Autodesk Fusion 360 part; units mm, degrees
sketch "Sketch1" plane through (0, 0, 0) normal (0, 1, 0) x (1, 0, 0)
  circle A0 centre (0, 0) radius 10.5
  dimension "d1" = 21
extrude "Extrude1" add sketch "Sketch1" along normal blind 4
sketch "Sketch2" plane through (0, 4, 0) normal (0, 1, 0) x (-1, 0, 0)
  circle A0 centre (0, 0) radius 10.5
  circle A1 centre (0, 0) radius 1.5
  dimension "d4" = 3
extrude "Extrude2" cut sketch "Sketch2" against normal blind 0.5 contours A1
sketch "Sketch3" plane through (0, 4, 0) normal (0, 1, 0) x (-1, 0, 0)
  circle A0 centre (0, 0) radius 1.5
  circle A1 centre (0, 0) radius 10.5
  circle A2 centre (0, 0) radius 9
  circle A3 centre (0, 0) radius 3.75
  dimension "d7" = 1.5
  dimension "d20" = 7.5
extrude "Extrude3" cut sketch "Sketch3" against normal blind 0.25
fillet "Fillet1" radius 0.1 1 edges at (-9.7894, 3.75, -3.797)
ref_plane "WorkPlane1" through (0, 0, 10.5) normal (0, 0, 1) x (1, 0, 0)
sketch "Sketch4" plane through (0, 0, 10.5) normal (0, 0, 1) x (1, 0, 0)
  line L0 (-1, 0) -> (1, 0)
  line L1 (1, 0) -> (1, 1.5)
  line L2 (1, 1.5) -> (-1, 1.5)
  line L3 (-1, 1.5) -> (-1, 0)
  line L4 (10.5, 0) -> (-10.5, 0)
  dimension "d12" = 1.5
  dimension "d13" = 2
extrude "Extrude4" cut sketch "Sketch4" against normal blind 0.5
sketch "Sketch5" plane through (0, 0, 10) normal (0, 0, 1) x (1, 0, 0)
  line L0 (1, 0) -> (1, 1.5)
  line L1 (1, 1.5) -> (-1, 1.5)
  line L2 (-1, 1.5) -> (-1, 0)
  line L3 (-1, 0) -> (1, 0)
  line L4 (9, 4) -> (-9, 4)
  line L5 (0, 1.5) -> (0, 0) construction
  line L6 (0, 0.75) -> (-1, 0.75) construction
  circle A0 centre (-0.5, 0.75) radius 0.25
  circle A1 centre (0.5, 0.75) radius 0.25
  dimension "d16" = 0.5
extrude "Extrude5" add sketch "Sketch5" along normal blind 2 contours A0 | A1
Part model, mm, in its own coordinate system. A direction names the side the tool comes from. Round coordinates to 2 decimals unless told otherwise and drop trailing zeros. Loops run counter-clockwise (first coordinate to the right, second up) from the corner with the lowest first, then second, coordinate; pieces in that order, holes last. Notation, with made-up numbers: (29, -27.75) - (40, -27.75) arc R13 ccw to (40, -14.75) - close; hole circle Ø5 at (21.25, 55.5). An arc over 180 degrees is marked (long way). Answer as a JSON object with one key per item and string values.
Item 1: Band-saw the part on B-B on x = 0. List the corners of the cut face in (y, z).
Output:
{"outline": "(0, -10.5) - (3.65, -10.5) arc R0.1 ccw to (3.75, -10.4) - (3.75, -9) - (4, -9) - (4, -3.75) - (3.75, -3.75) - (3.75, -1.5) - (3.5, -1.5) - (3.5, 1.5) - (3.75, 1.5) - (3.75, 3.75) - (4, 3.75) - (4, 9) - (3.75, 9) - (3.75, 10.4) arc R0.1 ccw to (3.65, 10.5) - (1.5, 10.5) - (1.5, 10) - (0, 10) - close"}
Item 2: Tool access for faces 1 (the face through (0, 3.5, 0)), 2 (the face through (0, 0, 0)), 3 (the face through (0, 1, 10)): list every direction of +Z, -Z, +X, -X, +Y, -Y with a clear straight run to the whole face (end or side of a thin tool).
Output:
{"face 1": "+Y", "face 2": "+Z, -Z, +X, -X, -Y", "face 3": "+Z"}
Item 3: Band-saw the part on A-A on y = 0.75. List the corners of the cut face in (x, z).
Output:
{"outline": "(-1, 10) - (-1, 10.45) arc R10.5 ccw (long way) to (1, 10.45) - (1, 10) - (0.75, 10) - (0.75, 12) - (0.25, 12) - (0.25, 10) - (-0.25, 10) - (-0.25, 12) - (-0.75, 12) - (-0.75, 10) - close"}
Item 4: Pull direction Z, two halves, no side cores. Call faces 4 (the face through (5, 3.75, 8)), 5 (the face through (0, 3.75, -2)), 6 (the face through (10, 1.8, 3.2)): pulls with the +Z half, pulls with the -Z half, needs draft (parallel to the pull), parting line crosses it, or undercut.
Output:
{"face 4": "needs draft", "face 5": "undercut", "face 6": "parting line crosses it"}
Item 5: Wall check: L1, parallel to Z at x = 0, y = 3.9; L2, parallel to Z at x = 0, y = 3.6; L3, parallel to Y at x = -1.25, z = 2.25. Give the ranges that are in metal, low to high.
Output:
{"L1": "-9 to -3.75, 3.75 to 9", "L2": "-10.5 to -1.5, 1.5 to 10.5", "L3": "0 to 3.75"}
Item 6: Pin check, flat tips, straight feed: pin 1 (1.5 mm diameter, centred on x = 7.5, y = 1, fed in from +Z); pin 2 (4 mm diameter, centred on x = -0.5, z = 1, fed in from +Y). Stop position of each tip, or through.
Output:
{"pin 1": "z = 8.04", "pin 2": "y = 3.75"}
Item 7: Band-saw the part on D-D on y = 2. List the corners of the cut face in (x, z).
Output:
{"outline": "circle Ø21 at (0, 0)"}
Item 8: Band-saw the part on C-C on z = 0. List the corners of the cut face in (x, y).
Output:
{"outline": "(-10.5, 0) - (10.5, 0) - (10.5, 3.65) arc R0.1 ccw to (10.4, 3.75) - (9, 3.75) - (9, 4) - (3.75, 4) - (3.75, 3.75) - (1.5, 3.75) - (1.5, 3.5) - (-1.5, 3.5) - (-1.5, 3.75) - (-3.75, 3.75) - (-3.75, 4) - (-9, 4) - (-9, 3.75) - (-10.4, 3.75) arc R0.1 ccw to (-10.5, 3.65) - close"}
